```python
from build123d import *

# Parameters (mm, degrees)
F0_W     = 60
F0_H     = 10
F1_DEPTH = 8
F2_DEPTH = 8
F3_W     = 10
F3_H     = 25
F3_W_2   = 25
F3_H_2   = 10
F4_DEPTH = 3
F5_DEPTH = 16


with BuildPart() as f1:
    # F0 (on Right) → F1 (new body)
    with BuildSketch(Plane.YZ):
        with Locations((0, 5)):
            Rectangle(F0_W, F0_H)
        Polygon((-30, 70), (-30, 10), (30, 10), (30, 70), (20, 70), (20, 30), (-20, 30), (-20, 70), align=None)
    extrude(amount=-F1_DEPTH)

    # F0 (on Right) → F2 (join)
    with BuildSketch(Plane.YZ):
        with Locations((0, 5)):
            Rectangle(F0_W, F0_H)
    extrude(amount=F2_DEPTH)

    # F3 (on face) → F4 (cut)
    with BuildSketch(Plane(origin=(-8, 0, 0), x_dir=(0, -1, 0), z_dir=(-1, 0, 0))):
        with Locations((-25, 52.5)):
            Rectangle(F3_W, F3_H)
        with Locations((25, 52.5)):
            Rectangle(F3_W, F3_H)
        with Locations((0, 25)):
            Rectangle(F3_W_2, F3_H_2)
    extrude(amount=-F4_DEPTH, mode=Mode.SUBTRACT)

    # F0 (on Right) → F5 (join)
    with BuildSketch(Plane.YZ):
        with Locations((0, 5)):
            Rectangle(F0_W, F0_H)
    extrude(amount=-F5_DEPTH)


solid = f1.part
```
The listing builds one solid part. Answer for the finished solid, in the listing's coordinates (mm). A direction names the side the tool comes from. Coordinates: 2 decimals unless noted, no trailing zeros. Write each loop counter-clockwise with the first axis right and the second up, starting at its lowest first coordinate (ties: lowest second). Pieces come first, ordered by that corner, then holes.
Q1. The mould has two halves that part along Z. Classify faces 5 (the flat face through (-3, 0, 30)), 6 (the flat face through (-7, -25, 65)), 7 (the flat face through (-4, 0, 0)), 8 (the flat face through (-4, -30, 27)): released by +Z, released by -Z, zero draft, split by the parting line, or undercut.
Returned:
face 5: released by +Z
face 6: undercut
face 7: released by -Z
face 8: zero draft
Q2. Section D-D, the plane x = 1 is taken. Write down the section's boundary in (y, z), then the cut area to 3 significant figures.
Returned:
outline: (-30, 0) - (30, 0) - (30, 10) - (-30, 10) - close
area: 600 mm2
Q3. Section C-C, the plane z = 25.5 is taken. Write down the section's boundary in (x, y), then the cut area to 3 significant figures.
Returned:
outline: (-8, -30) - (0, -30) - (0, 30) - (-8, 30) - (-8, 12.5) - (-5, 12.5) - (-5, -12.5) - (-8, -12.5) - close
area: 405 mm2
Q4. Section A-A, the plane z = 61 is taken. Write down the section's boundary in (x, y).
Returned:
outline: (-5, -30) - (0, -30) - (0, -20) - (-5, -20) - close; (-5, 20) - (0, 20) - (0, 30) - (-5, 30) - close
Q5. Section B-B, the plane y = 7 is taken. Write down the section's boundary in (x, z), then the cut area to 3 significant figures.
Returned:
outline: (-16, 0) - (8, 0) - (8, 10) - (0, 10) - (0, 30) - (-5, 30) - (-5, 20) - (-8, 20) - (-8, 10) - (-16, 10) - close
area: 370 mm2
Q6. Which of the six approach directions +Z, -Z, +X, -X, +Y, -Y give full straight-line access (tool end or side, diameter ignored) to faces 1 (the flat face through (-8, -25, 68)), 2 (the flat face through (-7, 0, 20)), 3 (the flat face through (-5, 25, 53)), 4 (the flat face through (4, 0, 10))?
Returned:
face 1: +Z, -X, +Y, -Y
face 2: +Z, -X
face 3: -X, +Y, -Y
face 4: +Z, +X, +Y, -Y
Q7. Given P1, Ø6.5, axis at x = -11, y = 6, coming from the +Z side; P2, Ø6, axis at y = -20, z = 42, coming from the -X side; P3, Ø9, axis at x = 3.5, y = 7.5, coming from the +Z side; P4, Ø0.9, axis at x = -6, y = 26.5, coming from the -Z side, each flat-ended and moving along its own axis, determine where each tip first touches the part or whether it passes through.
Returned:
P1: stops at z = 20
P2: stops at x = -8
P3: stops at z = 30
P4: stops at z = 0
Q8. Find the intervals of material crossed by line 1 along Y through (x, z) = (-7.75, 36.5); line 2 along Z through (x, y) = (-6, -25); line 3 along Z through (x, y) = (-11.25, -17), in increasing order.
Returned:
line 1: y = -30 to -20, 20 to 30
line 2: z = 0 to 40, 65 to 70
line 3: z = 0 to 10
